Autodesk Inventor part; units mm, degrees
ref_plane "YZ Plane" through (0, 0, 0) normal (1, 0, 0) x (0, 1, 0)
ref_plane "XZ Plane" through (0, 0, 0) normal (0, 1, 0) x (-1, 0, 0)
ref_plane "XY Plane" through (0, 0, 0) normal (0, 0, 1) x (1, 0, 0)
sketch "Sketch1" plane through (0, 0, 0) normal (0, 0, 1) x (1, 0, 0)
  line L0 (0, 0) -> (120, 0)
  arc A0 (0, 3) -> (0, 0) centre (0, 1.5) ccw
  arc A1 (120, 0) -> (120, 3) centre (120, 1.5) ccw
  circle A2 centre (0, 1.5) radius 1
  circle A3 centre (120, 1.5) radius 1
  arc A4 (75.9569, 30.1419) -> (74.6624, 30.2712) centre (75.1754, 28.8616) ccw
  line L1 (53.292, 22.493) -> (62.7991, 25.9533)
  line L2 (62.7991, 25.9533) -> (74.6624, 30.2712)
  line L3 (53.292, 22.493) -> (-0.513, 2.9095)
  line L4 (80.4155, 27.4204) -> (88.5179, 22.4745)
  line L5 (80.4155, 27.4204) -> (75.9569, 30.1419)
  line L6 (88.5179, 22.4745) -> (120.7815, 2.7803)
  dimension "d0" = 2
  dimension "d1" = 2
  dimension "d2" = 120
  dimension "d8" = 3
extrude "Extrusion1" add sketch "Sketch1" along normal blind 3
properties part number "L3"
Model file for the job. Use its own axes, mm. Give positions to 0.01 mm unless a question says otherwise; leave off trailing zeros. Loops run counter-clockwise (first coordinate to the right, second up) from the corner with the lowest first, then second, coordinate; pieces in that order, holes last. Notation, with made-up numbers: (60.25, 74) - (118.25, 74) arc R19 cw to (118.25, 108) - close; hole circle Ø10 at (6.5, -16). An arc over 180 degrees is marked (long way). Use one line per item in the form item = value.
(1) Cut at A-A (z = 1.4). Give the cut face in (x, y), then the cut area to 3 significant figures.
Determined:
outline = (-0.51, 2.91) arc R1.5 ccw to (0, 0) - (120, 0) arc R1.5 ccw to (120.78, 2.78) - (88.52, 22.47) - (80.42, 27.42) - (75.96, 30.14) arc R1.5 ccw to (74.66, 30.27) - (62.8, 25.95) - (53.29, 22.49) - close; hole circle Ø2 at (0, 1.5); hole circle Ø2 at (120, 1.5)
area = 2,020 mm^2
(2) Cut at C-C (x = 97). Give the cut face in (y, z).
Determined:
outline = (0, 0) - (17.3, 0) - (17.3, 3) - (0, 3) - close
(3) Pull direction X, two halves, no side cores. Call faces 1 (the face through (121.45, 1.12, 1.48)), 2 (the face through (-0.217, 2.476, 1.479)), 3 (the face through (-1.47, 1.21, 1.48)), 4 (the face through (119, 1.5, 1.5)): pulls with the +X half, pulls with the -X half, needs draft (parallel to the pull), parting line crosses it, or undercut.
Determined:
face_1 = pulls with the +X half
face_2 = undercut
face_3 = pulls with the -X half
face_4 = undercut
(4) Drill centre lines: L1, parallel to Y at x = 0, z = 2.4; L2, parallel to Y at x = 85, z = 0.75; L3, parallel to Y at x = 28.5, z = 1.65. Where is each one in solid material? Low to high.
Determined:
L1 = 0 to 0.5, 2.5 to 3.1
L2 = 0 to 24.62
L3 = 0 to 13.47
(5) Cut at B-B (y = 14). Give the cut face in (x, z), then the cut area to 3 significant figures.
Determined:
outline = (29.96, 0) - (102.4, 0) - (102.4, 3) - (29.96, 3) - close
area = 217 mm^2
